from build123d import *

# Parameters (mm, degrees)
SKETCH1_W               = 60
SKETCH1_H               = 60
BOSS_EXTRUDE1_DEPTH     = 40
SKETCH2_R               = 2.5
CUT_EXTRUDE1_DEPTH      = 65.031242374
FILLET1_R               = 4
FILLET2_R               = 1
CUT_EXTRUDE2_DEPTH      = 66.946948375
CUT_EXTRUDE2_DEPTH_BACK = 66.946948375
SKETCH5_W               = 2.5
SKETCH5_H               = 27


with BuildPart() as part:
    # Sketch1 → Boss-Extrude1 (new body)
    with BuildSketch(Plane(origin=(-3, 0, 0), x_dir=(0, 0, -1), z_dir=(1, 0, 0))):
        with Locations((0, -10)):
            Rectangle(SKETCH1_W, SKETCH1_H)
    extrude(amount=-BOSS_EXTRUDE1_DEPTH)

    # Sketch2 → Cut-Extrude1 (cut, through all)
    with BuildSketch(Plane(origin=(-3, 0, 0), x_dir=(0, 0, -1), z_dir=(1, 0, 0))):
        with Locations((-24.747474619, 14.75)):
            Circle(SKETCH2_R)
        with Locations((24.747474619, 14.75)):
            Circle(SKETCH2_R)
        with Locations((24.747474619, -34.75)):
            Circle(SKETCH2_R)
        with Locations((-24.747474619, -34.75)):
            Circle(SKETCH2_R)
    extrude(amount=-CUT_EXTRUDE1_DEPTH, mode=Mode.SUBTRACT)

    # Fillet1
    fillet1_edges = [part.edges().sort_by_distance(p)[0] for p in [
        (-23, 20, 30),
        (-23, 20, -30),
        (-23, -40, -30),
        (-23, -40, 30),
    ]]
    fillet(fillet1_edges, radius=FILLET1_R)

    # Sketch3 → Revolve1 (revolve)
    with BuildSketch(Plane.XY, mode=Mode.PRIVATE) as revolve1_sk:
        Polygon((-3, 12), (0, 12), (0, 4), (29.2, 4), (29.2, 0), (-3, 0), align=None)
    revolve(revolve1_sk.sketch.rotate(Axis((-3, 0, 0), (1, 0, 0)), 90), axis=Axis((-3, 0, 0), (1, 0, 0)))

    # Fillet2
    fillet2_edges = [part.edges().sort_by_distance(p)[0] for p in [
        (0, 0, -12),
        (29.2, 0, -4),
    ]]
    fillet(fillet2_edges, radius=FILLET2_R)

    # Sketch4 → Cut-Extrude2 (cut, two sides: drawn at the far end of the back side and taken through both)
    with BuildSketch(Plane.XY.offset(-CUT_EXTRUDE2_DEPTH_BACK)):
        with BuildLine():
            Line((29.2, 4), (9.2, 4))
            ThreePointArc((9.2, 4), (10.784573983, 3.255437353), (12.51662479, 3))
            Line((12.51662479, 3), (29.2, 3))
            Line((29.2, 3), (29.2, 4))
        make_face()
    extrude(amount=CUT_EXTRUDE2_DEPTH + CUT_EXTRUDE2_DEPTH_BACK, mode=Mode.SUBTRACT)

    # Sketch5 → Cut-Revolve1 (revolve, cut)
    with BuildSketch(Plane.XY, mode=Mode.PRIVATE) as cut_revolve1_sk:
        with Locations((-41.75, 3.5)):
            Rectangle(SKETCH5_W, SKETCH5_H)
    revolve(cut_revolve1_sk.sketch.rotate(Axis((-40.5, -10, 0), (-1, 0, 0)), 90), axis=Axis((-40.5, -10, 0), (-1, 0, 0)), mode=Mode.SUBTRACT)


solid = part.part
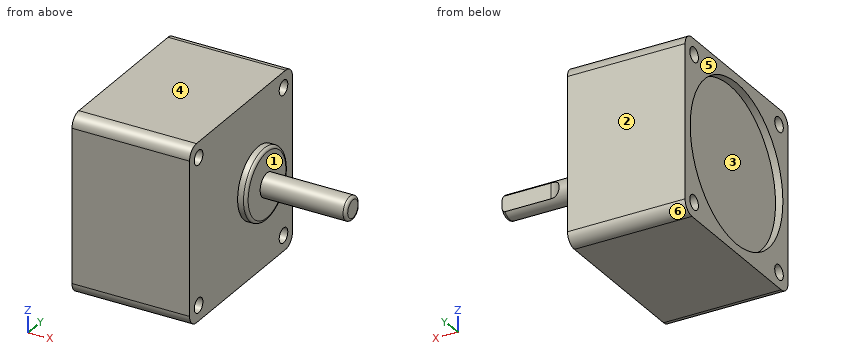
Part model, mm, in its own coordinate system. Face numbers are marked on the shaded views. A direction names the side the tool comes from. Round coordinates to 2 decimals unless told otherwise and drop trailing zeros. Order: outer loops, then holes, each group sorted by start corner. A loop starts at its lowest first (then second) coordinate and runs counter-clockwise, first axis right, second up. Notation, with made-up numbers: (52.5, -26) -> (59.5, -26) arc R12 cw to (59.5, -18) -> close; hole circle Ø5 at (-1, 36.5). An arc over 180 degrees is marked (long way). Put each result on its own line as item: value.
Q1. Pull direction Z, two halves, no side cores. Call the marked faces 3, 4, 5 and 6: pulls with the +Z half, pulls with the -Z half, needs draft (parallel to the pull), parting line crosses it, or undercut.
From the geometry:
face 3: undercut
face 4: pulls with the +Z half
face 5: needs draft
face 6: pulls with the -Z half
Q2. Band-saw the part on A-A (x = -18.5). Give the cut face in (y, z), and give its area (3 significant figures).
From the geometry:
outline: (-40, -26) arc R4 ccw to (-36, -30) -> (16, -30) arc R4 ccw to (20, -26) -> (20, 26) arc R4 ccw to (16, 30) -> (-36, 30) arc R4 ccw to (-40, 26) -> close; hole circle Ø5 at (-34.75, -24.75); hole circle Ø5 at (-34.75, 24.75); hole circle Ø5 at (14.75, -24.75); hole circle Ø5 at (14.75, 24.75)
area: 3,510 mm2
Q3. Band-saw the part on D-D (y = 0). Give the cut face in (x, z).
From the geometry:
outline: (-43, -30) -> (-3, -30) -> (-3, -12) -> (-1, -12) arc R1 ccw to (0, -11) -> (0, -4) -> (28.2, -4) arc R1 ccw to (29.2, -3) -> (29.2, 3) arc R1 ccw to (28.2, 4) -> (0, 4) -> (0, 11) arc R1 ccw to (-1, 12) -> (-3, 12) -> (-3, 30) -> (-43, 30) -> (-43, 25.08) -> (-40.5, 25.08) -> (-40.5, -25.08) -> (-43, -25.08) -> close
Q4. Wall check: line 1 (Y direction, x = -6.5, z = -24.5); line 2 (Z direction, x = -25, y = -34); line 3 (Y direction, x = -20, z = -23). Give the ranges that are in metal, low to high. Write a range as [from, to].
From the geometry:
line 1: y = [-40, -37.24], [-32.26, 12.26], [17.24, 20]
line 2: z = [-30, -27.13], [-22.36, 22.36], [27.13, 30]
line 3: y = [-40, -36.54], [-32.96, 12.96], [16.54, 20]
Q5. Tool access for the marked faces 1 and 2: list every direction of +Z, -Z, +X, -X, +Y, -Y with a clear straight run to the whole face (end or side of a thin tool).
From the geometry:
face 1: +X
face 2: +Z, -Z, +X, -X, +Y
Q6. Pin check, flat tips, straight feed: pin 1 Ø8 at (y, z) = (14.75, -24.75) entering from +X; pin 2 Ø5 at (y, z) = (-0.5, 7) entering from -X; pin 3 Ø2.5 at (x, z) = (20, -1) entering from +Y. Stop position of each tip, or through.
From the geometry:
pin 1: stops at x = -3
pin 2: stops at x = -40.5
pin 3: stops at y = 3
Q7. Band-saw the part on C-C (z = -16). Give the cut face in (x, y), and give its area (3 significant figures).
From the geometry:
outline: (-43, -40) -> (-3, -40) -> (-3, 20) -> (-43, 20) -> (-43, 11.75) -> (-40.5, 11.75) -> (-40.5, -31.75) -> (-43, -31.75) -> close
area: 2,290 mm2
Q8. Band-saw the part on B-B (y = 14.75). Give the cut face in (x, z), and give its area (3 significant figures).
From the geometry:
outline: (-43, -30) -> (-3, -30) -> (-3, -27.25) -> (-43, -27.25) -> close; (-43, -22.25) -> (-3, -22.25) -> (-3, 22.25) -> (-43, 22.25) -> (-43, 10.79) -> (-40.5, 10.79) -> (-40.5, -10.79) -> (-43, -10.79) -> close; (-43, 27.25) -> (-3, 27.25) -> (-3, 30) -> (-43, 30) -> close
area: 1,950 mm2
